For this review, take the finished solid that the model builds, in its own axes (mm). A direction names the side the tool comes from. Coordinates: 2 decimals unless noted, no trailing zeros. Loops run counter-clockwise (first coordinate to the right, second up) from the corner with the lowest first, then second, coordinate; pieces in that order, holes last. Notation, with made-up numbers: (-32.75, -35) -> (-12.75, -35) arc R16 cw to (-12.75, -19) -> close; hole circle Ø1 at (33.5, 76). An arc over 180 degrees is marked (long way). One line per item, written item: value.
from build123d import *

# Parameters (mm, degrees)
EXTRUDE_1_DEPTH = 2.7
SKETCH_1_4_R    = 2.5
EXTRUDE_3_DEPTH = 0.9
EXTRUDE_START   = -0.9
SKETCH_1_3_R    = 2.5
SKETCH_1_3_R_2  = 1.65
EXTRUDE_2_DEPTH = 2


with BuildPart() as part:
    # 草图1 → 凸台-拉伸1 (new body)
    with BuildSketch(Plane(origin=(0, 0, 0), x_dir=(1, 0, 0), z_dir=(0, 1, 0))):
        Polygon((1.270170592, 0), (0.635085296, 1.1), (-0.635085296, 1.1), (-1.270170592, 0), (-0.635085296, -1.1), (0.635085296, -1.1), align=None)
    extrude(amount=EXTRUDE_1_DEPTH)

    # 草图1<4> → 凸台-拉伸3 (add)
    with BuildSketch(Plane(origin=(0, 0, 0), x_dir=(1, 0, 0), z_dir=(0, 1, 0))):
        with Locations(Location((0, 0, 0), (0, 0, 270))):
            Circle(SKETCH_1_4_R)
    extrude(amount=-EXTRUDE_3_DEPTH)

    # 草图1<3> → 凸台-拉伸2 (add)
    # profile 1 of 3: a face of its own
    with BuildSketch(Plane(origin=(0, 0, 0), x_dir=(1, 0, 0), z_dir=(0, 1, 0)).offset(EXTRUDE_START)):
        with Locations(Location((0, 0, 0), (0, 0, 270))):
            Circle(SKETCH_1_3_R)
        Circle(SKETCH_1_3_R_2, mode=Mode.SUBTRACT)
    # profile 2 of 3: a face of its own
    with BuildSketch(Plane(origin=(0, 0, 0), x_dir=(1, 0, 0), z_dir=(0, 1, 0)).offset(EXTRUDE_START)):
        with BuildLine():
            ThreePointArc((1.65, 0), (1.478597308, 0.732290926), (1, 1.312440475))
            Line((1, 1.312440475), (1, 0.467949192))
            Line((1, 0.467949192), (1.270170592, 0))
            Line((1.270170592, 0), (1, -0.467949192))
            Line((1, -0.467949192), (1, -1.312440475))
            ThreePointArc((1, -1.312440475), (1.478597308, -0.732290926), (1.65, 0))
        make_face()
    # profile 3 of 3: a face of its own
    with BuildSketch(Plane(origin=(0, 0, 0), x_dir=(1, 0, 0), z_dir=(0, 1, 0)).offset(EXTRUDE_START)):
        Polygon((1.270170592, 0), (1, 0.467949192), (1, -0.467949192), align=None)
    extrude(amount=-EXTRUDE_2_DEPTH)


solid = part.part
1. Take a section at D-D, the plane y = -1.75. Give the boundary of the cut face in (x, z).
Return value:
outline: circle Ø5 at (0, 0); hole (1, -1.31) -> (1, 1.31) arc R1.65 ccw (long way) to start
2. For faces 4 (the cylindrical face through (-1.65, -1.89, -0.05)), 5 (the flat face through (0, 1, -1.1)), 6 (the flat face through (0.96, 1.33, -0.54)), list the 3-axis set-ups (+Z, -Z, +X, -X, +Y, -Y) from which the entire face can be reached by the end or side of a thin tool; tool diameter is ignored.
Return value:
face 4: -Y
face 5: -Z, +X, -X, +Y
face 6: -Z, +X, +Y
3. Insertion check: pin 1 Ø2.5 at (x, z) = (1, -1) entering from +Y; pin 2 Ø3 at (x, y) = (2, 2) entering from +Z; pin 3 Ø1 at (x, y) = (0, 1.5) entering from -Z; pin 4 Ø0.6 at (y, z) = (-1.5, -0.5) entering from -X. Each pin has a flat end and moves straight along its axis. Give the tip position at first contact, or say it passes through.
Return value:
pin 1: stops at y = 2.7
pin 2: stops at z = 1.1
pin 3: stops at z = -1.1
pin 4: stops at x = -2.49
4. Take a section at B-B, the plane y = 2.05. Give the boundary of the cut face in (x, z).
Return value:
outline: (-1.27, 0) -> (-0.64, -1.1) -> (0.64, -1.1) -> (1.27, 0) -> (0.64, 1.1) -> (-0.64, 1.1) -> close
5. Take a section at A-A, the plane x = 0. Give the boundary of the cut face in (y, z), and give its area (3 significant figures).
Return value:
outline: (-2.9, -2.5) -> (0, -2.5) -> (0, -1.1) -> (2.7, -1.1) -> (2.7, 1.1) -> (0, 1.1) -> (0, 2.5) -> (-2.9, 2.5) -> (-2.9, 1.65) -> (-0.9, 1.65) -> (-0.9, -1.65) -> (-2.9, -1.65) -> close
area: 13.8 mm2
6. The part is to be moulded in two halves that separate along Z. For faces 1 (the flat face through (0, 1, 1.1)), 2 (the flat face through (0, -0.9, 0)), 3 (the flat face through (-1, 0, 1)), say which applies: pulls with the +Z half, pulls with the -Z half, needs draft (parallel to the pull), parting line crosses it, or undercut.
Return value:
face 1: pulls with the +Z half
face 2: undercut
face 3: needs draft
7. Take a section at C-C, the plane z = -1.4. Give the boundary of the cut face in (x, y).
Return value:
outline: (-2.07, -2.9) -> (-0.87, -2.9) -> (-0.87, -0.9) -> (0.87, -0.9) -> (0.87, -2.9) -> (2.07, -2.9) -> (2.07, 0) -> (-2.07, 0) -> close
8. To check wall thickness, follow probe 1 along X at (y, z) = (-1.4, 0); probe 2 along Y at (x, z) = (0, -1); probe 3 along Y at (x, z) = (-1.45, -1.75). State the ranges of each line that lie inside material, in increasing order. Write a range as from..to.
Return value:
probe 1: x = -2.5..-1.65, 1..2.5
probe 2: y = -0.9..2.7
probe 3: y = -2.9..0
